```python
from build123d import *

# Parameters (mm, degrees)
CUT_EXTRUDE3_START         = -17.750008032
CUT_EXTRUDE3_OUTLINE_W     = 3.00000608
CUT_EXTRUDE3_OUTLINE_H     = 30.000001192
CUT_EXTRUDE3_OUTLINE_W_2   = 2.999998629
CUT_EXTRUDE3_DEPTH         = 17.750008032
CUT_EXTRUDE3_2_OUTLINE_W   = 9.999990463
CUT_EXTRUDE3_2_OUTLINE_H   = 30.000001192
CUT_EXTRUDE3_2_OUTLINE_W_2 = 10.000005364
CUT_EXTRUDE3_2_DEPTH       = 3.000000026
CUT_EXTRUDE3_START_2       = -3.000000492
CUT_EXTRUDE3_3_OUTLINE_W   = 12.49999553
CUT_EXTRUDE3_3_OUTLINE_H   = 30.000001192
CUT_EXTRUDE3_3_DEPTH       = 3.000000492
CUT_EXTRUDE3_START_3       = 85.588127375
CUT_EXTRUDE3_4_DEPTH       = 30.000001192
SKETCH7_W                  = 9
SKETCH7_H                  = 9
SKETCH11_W                 = 16.000001486
SKETCH11_H                 = 9
BOSS_EXTRUDE5_DEPTH        = 4
SKETCH12_W                 = 20.155891034
SKETCH12_H                 = 17
BOSS_EXTRUDE6_DEPTH        = 4
CUT_EXTRUDE4_DEPTH         = 20
CUT_EXTRUDE4_DEPTH_BACK    = 20
SKETCH13_W                 = 17.750008032
SKETCH13_H                 = 30.000001192


with BuildPart() as part:
    # Cut-Extrude3: read off the stored shape, not the designer's step
    # Cut-Extrude3 outline → Cut-Extrude3 (new body)
    with BuildSketch(Plane.XY.offset(17.750008032).offset(CUT_EXTRUDE3_START)):
        with Locations((137.970902026, 100.588127971)):
            Rectangle(CUT_EXTRUDE3_OUTLINE_W, CUT_EXTRUDE3_OUTLINE_H)
        with Locations((122.470904142, 100.588127971)):
            Rectangle(CUT_EXTRUDE3_OUTLINE_W_2, CUT_EXTRUDE3_OUTLINE_H)
    extrude(amount=CUT_EXTRUDE3_DEPTH)

    # Cut-Extrude3 2 outline → Cut-Extrude3 2 (add)
    # profile 1 of 2: a face of its own
    with BuildSketch(Plane.XY.offset(17.750008032).offset(CUT_EXTRUDE3_START)):
        with Locations((144.470900298, 100.588127971)):
            Rectangle(CUT_EXTRUDE3_2_OUTLINE_W, CUT_EXTRUDE3_2_OUTLINE_H)
        Polygon((146.020904183, 100.58812052), (145.813241601, 99.813126028), (145.24589479, 99.245779216), (144.470900297, 99.038124084), (143.695905805, 99.245779216), (143.128573895, 99.813126028), (142.920896411, 100.58812052), (143.128573895, 101.363122463), (143.695905805, 101.930469275), (144.470900297, 102.138124406), (145.24589479, 101.930469275), (145.813241601, 101.363122463), align=None, mode=Mode.SUBTRACT)
    # profile 2 of 2: a face of its own
    with BuildSketch(Plane.XY.offset(17.750008032).offset(CUT_EXTRUDE3_START)):
        with Locations((115.970902145, 100.588127971)):
            Rectangle(CUT_EXTRUDE3_2_OUTLINE_W_2, CUT_EXTRUDE3_2_OUTLINE_H)
        Polygon((114.628560841, 101.363122463), (115.195907652, 101.930469275), (115.970902145, 102.138124406), (116.745904088, 101.930469275), (117.313250899, 101.363122463), (117.520906031, 100.58812052), (117.313250899, 99.813126028), (116.745904088, 99.245779216), (115.970902145, 99.038124084), (115.195907652, 99.245779216), (114.628560841, 99.813126028), (114.420905709, 100.58812052), align=None, mode=Mode.SUBTRACT)
    extrude(amount=CUT_EXTRUDE3_2_DEPTH)

    # Cut-Extrude3 3 outline → Cut-Extrude3 3 (add)
    with BuildSketch(Plane.XY.offset(17.750008032).offset(CUT_EXTRUDE3_START_2)):
        with Locations((130.220901221, 100.588127971)):
            Rectangle(CUT_EXTRUDE3_3_OUTLINE_W, CUT_EXTRUDE3_3_OUTLINE_H)
    extrude(amount=CUT_EXTRUDE3_3_DEPTH)

    # Cut-Extrude3 4 outline → Cut-Extrude3 4 (add)
    with BuildSketch(Plane(origin=(0, 0, 0), x_dir=(1, 0, 0), z_dir=(0, 1, 0)).offset(CUT_EXTRUDE3_START_3)):
        Polygon((139.738842845, -4.00000019), (140.470907092, -3.267952008), (141.470894217, -3.000000026), (139.470905066, -3.000000026), (139.470905066, -5.000007804), align=None)
        Polygon((118.970900774, -3.000000026), (119.970902801, -3.267952008), (120.702959597, -4.00000019), (120.970904827, -5.000007804), (120.970904827, -3.000000026), align=None)
    extrude(amount=CUT_EXTRUDE3_4_DEPTH)

    # Sweep1: sweep along a path in Sketch5
    with BuildLine(Plane(origin=(130.220903456, 0, 0), x_dir=(0, 0, -1), z_dir=(1, 0, 0))) as sweep1_path:
        Line((-17.750008032, 100.588127971), (-80.246052562, 100.588127971))
        Line((-80.246052562, 100.588127971), (-80.246052562, 57.588127971))
        Line((-80.246052562, 57.588127971), (-113.246052562, 57.588127971))
        Line((-113.246052562, 57.588127971), (-122.756617725, 60.678297914))
    # Sketch7 → Sweep1 (sweep)
    with BuildSketch(Plane.XY.offset(17.750008032)):
        with Locations((130.220904946, 100.588127971)):
            Rectangle(SKETCH7_W, SKETCH7_H)
    sweep(path=sweep1_path.line, transition=Transition.RIGHT)

    # Sketch11 → Boss-Extrude5 (add)
    with BuildSketch(Plane(origin=(0, 41.871526616, 128.867308142), x_dir=(1, 0, 0), z_dir=(0, 0.30901699437494257, 0.9510565162951552))):
        with Locations((126.720904203, 19.77460958)):
            Rectangle(SKETCH11_W, SKETCH11_H)
    extrude(amount=BOSS_EXTRUDE5_DEPTH)

    # Sketch12 → Boss-Extrude6 (add)
    with BuildSketch(Plane(origin=(0, 43.107594593, 132.671534207), x_dir=(1, 0, 0), z_dir=(0, 0.3090169943749432, 0.951056516295155))):
        with Locations((128.72090495, 19.77460958)):
            Rectangle(SKETCH12_W, SKETCH12_H)
    extrude(amount=BOSS_EXTRUDE6_DEPTH)

    # Sketch13 → Cut-Extrude4 (cut, two sides: drawn at the far end of the back side and taken through both)
    with BuildSketch(Plane(origin=(130.220903456, 0, 0), x_dir=(0, 0, -1), z_dir=(1, 0, 0)).offset(-CUT_EXTRUDE4_DEPTH_BACK)):
        with Locations((-8.875004016, 100.588127971)):
            Rectangle(SKETCH13_W, SKETCH13_H)
    extrude(amount=CUT_EXTRUDE4_DEPTH + CUT_EXTRUDE4_DEPTH_BACK, mode=Mode.SUBTRACT)


solid = part.part
```
Verification items for the finished model (mm, model axes). A direction names the side the tool comes from. Coordinates: 2 decimals unless noted, no trailing zeros. Order: outer loops, then holes, each group sorted by start corner. A loop starts at its lowest first (then second) coordinate and runs counter-clockwise, first axis right, second up. Notation, with made-up numbers: (-14.5, 15.25) -> (39.5, 15.25) arc R22 cw to (39.5, 25.25) -> close; hole circle Ø9 at (50.25, -20). An arc over 180 degrees is marked (long way). Answer as CSV lines item,"result". Start each with the question number.
1) Release check for a two-part mould opening along Z. For faces 1 (the face through (130, 105.088, 52)), 2 (the face through (130, 74, 75.746)), 3 (the face through (130, 62.088, 99)) record: released by +Z, released by -Z, zero draft, split by the parting line, or undercut.
2) Cross-section at C-C, the plane z = 70.5. Record the boundary of the cut face in (x, y).
3) Cross-section at B-B, the plane y = 78. Record the boundary of the cut face in (x, z), then the cut area to 3 significant figures.
4) Material ranges on L1, parallel to Y at x = 128.5, z = 91.5; L2, parallel to X at y = 98, z = 65; L3, parallel to Y at x = 131.5, z = 71, recorded low to high. Write a range as [from, to].
5) Set-up check for faces 4 (the face through (128.58, 70.608, 125.81)), 5 (the face through (130, 96.088, 47)), 6 (the face through (118.721, 61, 125)): record each of +Z, -Z, +X, -X, +Y, -Y from which the full face is reachable in a straight line by a thin tool's end or side.
6) Cross-section at D-D, the plane x = 123. Record the boundary of the cut face in (y, z).
7) Gauge pin test, flat ends, axial feed: pin 1 Ø2.5 at (x, z) = (130.5, 101) entering from +Y; pin 2 Ø2.5 at (x, y) = (130.5, 81) entering from -Z; pin 3 Ø2.5 at (x, y) = (131.5, 86) entering from +Z; pin 4 Ø7 at (y, z) = (60, 125) entering from -X. Record the tip position at first contact, or that the pin passes through.
8) Cross-section at A-A, the plane x = 129.75. Record the boundary of the cut face in (y, z), then the cut area to 3 significant figures.
Conclusion:
1,face 1,"zero draft"
1,face 2,"released by -Z"
1,face 3,"undercut"
2,outline,"(125.72, 96.09) -> (134.72, 96.09) -> (134.72, 105.09) -> (125.72, 105.09) -> close"
3,outline,"(125.72, 75.75) -> (134.72, 75.75) -> (134.72, 84.75) -> (125.72, 84.75) -> close"
3,area,"81.0 mm²"
4,L1,"y = [53.09, 62.09]"
4,L2,"x = [125.72, 134.72]"
4,L3,"y = [96.09, 105.09]"
5,face 4,"+X, -X, +Y"
5,face 5,"-Z, +X, -X, -Y"
5,face 6,"-Z, -X, -Y"
6,outline,"(53.83, 129.19) -> (57.63, 127.95) -> (56.4, 124.15) -> (64.96, 121.37) -> (66.19, 125.17) -> (70, 123.93) -> (71.23, 127.74) -> (55.07, 132.99) -> close"
7,pin 1,"stops at y = 62.09"
7,pin 2,"stops at z = 75.75"
7,pin 3,"stops at z = 84.75"
7,pin 4,"stops at x = 118.64"
8,outline,"(53.09, 75.75) -> (96.09, 75.75) -> (96.09, 17.75) -> (105.09, 17.75) -> (105.09, 84.75) -> (62.09, 84.75) -> (62.09, 112.53) -> (66.19, 125.17) -> (70, 123.93) -> (71.23, 127.74) -> (55.07, 132.99) -> (53.83, 129.19) -> (57.63, 127.95) -> (53.09, 113.96) -> close"
8,area,"1,440 mm²"
